Can you work these out from the model? Positions are in its coordinate system, mm. Face numbers are marked on the shaded views. Round coordinates to 2 decimals unless told otherwise and drop trailing zeros. Order: outer loops, then holes, each group sorted by start corner. A loop starts at its lowest first (then second) coordinate and runs counter-clockwise, first axis right, second up.
Q1. If I drill on line 1 (Y direction, x = 121, z = -60.5); line 2 (Z direction, x = 257.5, y = 70); line 3 (X direction, y = 78, z = -110.5), over which ranges is the centre line in solid material (lowest first)?
Q2. If we section it at D-D (z = -87.5): Please give me the cut outline in (x, y).
Q3. We'd pull the mould along X, two halves only. Please class the marked faces 1, 2, 3 and 4: pulls with the +X half, pulls with the -X half, needs draft (parallel to the pull), parting line crosses it, or undercut.
Q4. If we section it at A-A (z = -67): Please give me the cut outline in (x, y).
Q5. If we section it at C-C (x = 137): Please give me the cut outline in (y, z), plus the area to 3 significant figures.
Q6. Will this pin go through, and if not, where does the flat tip stop? P1, Ø8, axis at x = 72.5, y = 109, coming from the -Z side.
Q7. If we section it at B-B (y = 70): Please give me the cut outline in (x, z).
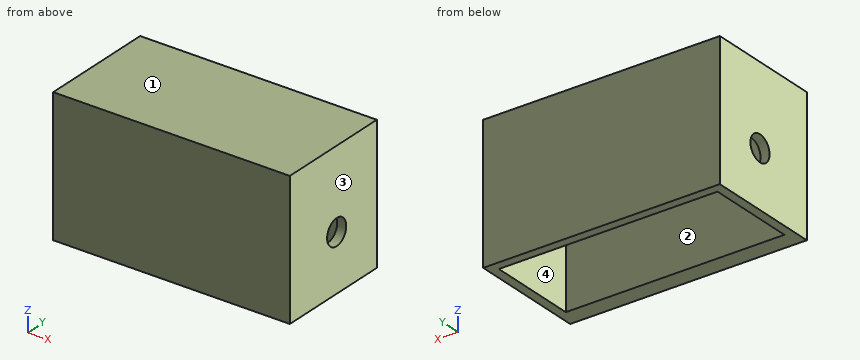
from build123d import *

# Parameters (mm, degrees)
SKETCH1_W           = 262
SKETCH1_H           = 150
BOSS_EXTRUDE1_DEPTH = 20
BOSS_EXTRUDE2_DEPTH = 100
SKETCH3_R           = 14.2875
CUT_EXTRUDE1_DEPTH  = 11
SKETCH4_R           = 14.2875
CUT_EXTRUDE2_DEPTH  = 11
SKETCH5_W           = 262
SKETCH5_H           = 150
BOSS_EXTRUDE4_DEPTH = 10


with BuildPart() as part:
    # Sketch1 → Boss-Extrude1 (new body)
    with BuildSketch(Plane(origin=(0, 0, 0), x_dir=(1, 0, 0), z_dir=(0, 1, 0))):
        with Locations((131, 75)):
            Rectangle(SKETCH1_W, SKETCH1_H)
    extrude(amount=BOSS_EXTRUDE1_DEPTH)

    # Sketch2 → Boss-Extrude2 (add)
    with BuildSketch(Plane(origin=(0, 20, 0), x_dir=(1, 0, 0), z_dir=(0, 1, 0))):
        Polygon((0, 0), (262, 0), (262, 150), (252, 150), (252, 10), (10, 10), (10, 150), (0, 150), align=None)
    extrude(amount=BOSS_EXTRUDE2_DEPTH)

    # Sketch3 → Cut-Extrude1 (cut, through all)
    with BuildSketch(Plane(origin=(10, 0, 0), x_dir=(0, 0, -1), z_dir=(1, 0, 0))):
        with Locations((87.5, 70)):
            Circle(SKETCH3_R)
    extrude(amount=-CUT_EXTRUDE1_DEPTH, mode=Mode.SUBTRACT)

    # Sketch4 → Cut-Extrude2 (cut, through all)
    with BuildSketch(Plane(origin=(252, 0, 0), x_dir=(0, 0, -1), z_dir=(1, 0, 0))):
        with Locations((87.5, 70)):
            Circle(SKETCH4_R)
    extrude(amount=CUT_EXTRUDE2_DEPTH, mode=Mode.SUBTRACT)

    # Sketch5 → Boss-Extrude4 (add)
    with BuildSketch(Plane(origin=(0, 120, 0), x_dir=(1, 0, 0), z_dir=(0, 1, 0))):
        with Locations((131, 75)):
            Rectangle(SKETCH5_W, SKETCH5_H)
    extrude(amount=BOSS_EXTRUDE4_DEPTH)


solid = part.part
Solution:
1. line 1: y = 0 to 20, 120 to 130
1. line 2: z = -150 to -101.79, -73.21 to 0
1. line 3: x = 0 to 10, 252 to 262
2. outline: (0, 0) - (262, 0) - (262, 55.71) - (252, 55.71) - (252, 20) - (10, 20) - (10, 55.71) - (0, 55.71) - close; (0, 84.29) - (10, 84.29) - (10, 120) - (252, 120) - (252, 84.29) - (262, 84.29) - (262, 130) - (0, 130) - close
3. face 1: needs draft
3. face 2: undercut
3. face 3: pulls with the +X half
3. face 4: undercut
4. outline: (0, 0) - (262, 0) - (262, 130) - (0, 130) - close; hole (10, 20) - (252, 20) - (252, 120) - (10, 120) - close
5. outline: (0, -150) - (20, -150) - (20, -10) - (120, -10) - (120, -150) - (130, -150) - (130, 0) - (0, 0) - close
5. area: 5,500 mm2
6. P1: stops at z = -10
7. outline: (0, -150) - (10, -150) - (10, -101.79) - (0, -101.79) - close; (0, -73.21) - (10, -73.21) - (10, -10) - (252, -10) - (252, -73.21) - (262, -73.21) - (262, 0) - (0, 0) - close; (252, -150) - (262, -150) - (262, -101.79) - (252, -101.79) - close
